```python
from build123d import *

# Parameters (mm, degrees)
BOSS_EXTRUDE1_DEPTH = 150


with BuildPart() as part:
    # Sketch1 → Boss-Extrude1 (new body)
    with BuildSketch(Plane.XY):
        with BuildLine():
            Line((12.999999999, 14.999999999), (10.499999999, 14.999999999))
            Line((10.499999999, 14.999999999), (9.999999999, 14.499999999))
            Line((9.999999999, 14.499999999), (9.5, 14.999999999))
            Line((9.5, 14.999999999), (4.5, 14.999999999))
            Line((4.5, 14.999999999), (4.5, 14.5))
            Line((4.5, 14.5), (4, 14.5))
            Line((4, 14.5), (4, 12.200000005))
            Line((4, 12.200000005), (7.999999994, 12.200000005))
            ThreePointArc((7.999999994, 12.200000005), (8.923879532, 11.582683434), (8.707106779, 10.492893215))
            Line((8.707106779, 10.492893215), (4.214213564, 6))
            Line((4.214213564, 6), (0.312520901, 6))
            Line((0.312520901, 6), (0, 5.7))
            Line((0, 5.7), (-0.312520903, 6))
            Line((-0.312520903, 6), (-4.214213564, 6))
            Line((-4.214213564, 6), (-8.70710678, 10.492893215))
            ThreePointArc((-8.70710678, 10.492893215), (-8.923879532, 11.582683434), (-7.999999995, 12.200000005))
            Line((-7.999999995, 12.200000005), (-4, 12.200000005))
            Line((-4, 12.200000005), (-4, 14.5))
            Line((-4, 14.5), (-4.5, 14.5))
            Line((-4.5, 14.5), (-4.5, 14.999999999))
            Line((-4.5, 14.999999999), (-9.500000003, 14.999999999))
            Line((-9.500000003, 14.999999999), (-10.000000002, 14.499999999))
            Line((-10.000000002, 14.499999999), (-10.500000001, 14.999999999))
            Line((-10.500000001, 14.999999999), (-13, 14.999999999))
            ThreePointArc((-13, 14.999999999), (-14.414213562, 14.414213561), (-15, 12.999999999))
            Line((-15, 12.999999999), (-15, 10.5))
            Line((-15, 10.5), (-14.500000001, 10.000000001))
            Line((-14.500000001, 10.000000001), (-15, 9.500000001))
            Line((-15, 9.500000001), (-15, 4.5))
            Line((-15, 4.5), (-14.5, 4.5))
            Line((-14.5, 4.5), (-14.5, 4))
            Line((-14.5, 4), (-12.200000005, 4))
            Line((-12.200000005, 4), (-12.200000005, 7.999999994))
            ThreePointArc((-12.200000005, 7.999999994), (-11.582683434, 8.923879532), (-10.492893215, 8.707106779))
            Line((-10.492893215, 8.707106779), (-6, 4.214213564))
            Line((-6, 4.214213564), (-6, 0.312520901))
            Line((-6, 0.312520901), (-5.7, 0))
            Line((-5.7, 0), (-6, -0.312520903))
            Line((-6, -0.312520903), (-6, -4.214213564))
            Line((-6, -4.214213564), (-10.492893215, -8.70710678))
            ThreePointArc((-10.492893215, -8.70710678), (-11.582683434, -8.923879532), (-12.200000005, -7.999999995))
            Line((-12.200000005, -7.999999995), (-12.200000005, -4))
            Line((-12.200000005, -4), (-14.5, -4))
            Line((-14.5, -4), (-14.5, -4.5))
            Line((-14.5, -4.5), (-15, -4.5))
            Line((-15, -4.5), (-15, -9.500000001))
            Line((-15, -9.500000001), (-14.500000001, -10.000000001))
            Line((-14.500000001, -10.000000001), (-15, -10.5))
            Line((-15, -10.5), (-15, -13))
            ThreePointArc((-15, -13), (-14.414213562, -14.414213562), (-13, -15))
            Line((-13, -15), (-10.489897949, -15))
            Line((-10.489897949, -15), (-9.989897949, -14.5))
            Line((-9.989897949, -14.5), (-9.500000001, -15))
            Line((-9.500000001, -15), (-4.5, -15))
            Line((-4.5, -15), (-4.5, -14.5))
            Line((-4.5, -14.5), (-4, -14.5))
            Line((-4, -14.5), (-4, -12.200000005))
            Line((-4, -12.200000005), (-7.999999995, -12.200000005))
            ThreePointArc((-7.999999995, -12.200000005), (-8.923879532, -11.582683434), (-8.70710678, -10.492893215))
            Line((-8.70710678, -10.492893215), (-4.214213564, -6))
            Line((-4.214213564, -6), (-0.312520901, -6))
            Line((-0.312520901, -6), (0, -5.7))
            Line((0, -5.7), (0.312520903, -6))
            Line((0.312520903, -6), (4.214213564, -6))
            Line((4.214213564, -6), (8.70710678, -10.492893215))
            ThreePointArc((8.70710678, -10.492893215), (8.923879532, -11.582683434), (7.999999995, -12.200000005))
            Line((7.999999995, -12.200000005), (4, -12.200000005))
            Line((4, -12.200000005), (4, -14.5))
            Line((4, -14.5), (4.5, -14.5))
            Line((4.5, -14.5), (4.5, -15))
            Line((4.5, -15), (9.500000001, -15))
            Line((9.500000001, -15), (10.000000001, -14.500000001))
            Line((10.000000001, -14.500000001), (10.5, -15))
            Line((10.5, -15), (12.999999999, -15))
            ThreePointArc((12.999999999, -15), (14.414213561, -14.414213562), (14.999999999, -13))
            Line((14.999999999, -13), (14.999999999, -10.500000001))
            Line((14.999999999, -10.500000001), (14.499999999, -10.000000002))
            Line((14.499999999, -10.000000002), (14.999999999, -9.500000002))
            Line((14.999999999, -9.500000002), (14.999999999, -4.5))
            Line((14.999999999, -4.5), (14.5, -4.5))
            Line((14.5, -4.5), (14.5, -4))
            Line((14.5, -4), (12.200000005, -4))
            Line((12.200000005, -4), (12.200000005, -7.999999995))
            ThreePointArc((12.200000005, -7.999999995), (11.582683434, -8.923879532), (10.492893215, -8.70710678))
            Line((10.492893215, -8.70710678), (6, -4.214213564))
            Line((6, -4.214213564), (6, -0.312520901))
            Line((6, -0.312520901), (5.7, 0))
            Line((5.7, 0), (6, 0.312520903))
            Line((6, 0.312520903), (6, 4.214213564))
            Line((6, 4.214213564), (10.492893215, 8.70710678))
            ThreePointArc((10.492893215, 8.70710678), (11.582683434, 8.923879532), (12.200000005, 7.999999995))
            Line((12.200000005, 7.999999995), (12.200000005, 4))
            Line((12.200000005, 4), (14.5, 4))
            Line((14.5, 4), (14.5, 4.5))
            Line((14.5, 4.5), (14.999999999, 4.5))
            Line((14.999999999, 4.5), (14.999999999, 9.5))
            Line((14.999999999, 9.5), (14.499999999, 9.999999999))
            Line((14.499999999, 9.999999999), (14.999999999, 10.499999999))
            Line((14.999999999, 10.499999999), (14.999999999, 12.999999999))
            ThreePointArc((14.999999999, 12.999999999), (14.414213561, 14.414213561), (12.999999999, 14.999999999))
        make_face()
        with BuildLine():
            Line((-2.902349714, 1.770978864), (-4.808326112, 3.676955262))
            Line((-4.808326112, 3.676955262), (-3.676955262, 4.808326112))
            Line((-3.676955262, 4.808326112), (-1.770978864, 2.902349714))
            ThreePointArc((-1.770978864, 2.902349714), (0, 3.4), (1.770978864, 2.902349714))
            Line((1.770978864, 2.902349714), (3.676955262, 4.808326112))
            Line((3.676955262, 4.808326112), (4.808326112, 3.676955262))
            Line((4.808326112, 3.676955262), (2.902349714, 1.770978864))
            ThreePointArc((2.902349714, 1.770978864), (3.4, 0), (2.902349714, -1.770978864))
            Line((2.902349714, -1.770978864), (4.808326112, -3.676955262))
            Line((4.808326112, -3.676955262), (3.676955262, -4.808326112))
            Line((3.676955262, -4.808326112), (1.770978864, -2.902349714))
            ThreePointArc((1.770978864, -2.902349714), (0, -3.4), (-1.770978864, -2.902349714))
            Line((-1.770978864, -2.902349714), (-3.676955262, -4.808326112))
            Line((-3.676955262, -4.808326112), (-4.808326112, -3.676955262))
            Line((-4.808326112, -3.676955262), (-2.902349714, -1.770978864))
            ThreePointArc((-2.902349714, -1.770978864), (-3.4, 0), (-2.902349714, 1.770978864))
        make_face(mode=Mode.SUBTRACT)
    extrude(amount=BOSS_EXTRUDE1_DEPTH)


solid = part.part
```
CAD build for the part. Positions are in the model's coordinates, mm. A direction names the side the tool comes from. Round coordinates to 2 decimals unless told otherwise and drop trailing zeros. One line per question, with ' | ' between items.
1. Probe L1, parallel to Y at x = -13, z = 27.5; L2, parallel to Y at x = -11.25, z = 45.5; L3, parallel to Y at x = -5, z = 138. List the from-to ranges inside material, lowest first. Write a range as from..to.
Working result:
L1: -15..-4, 4..15 | L2: -15..-9, 9..15 | L3: -15..-12.2, -6.79..6.79, 12.2..15
2. Mould opens along X. For faces 3 (the flat face through (-15, -12, 74)), 4 (the flat face through (2, 6, 74)), 5 (the flat face through (15, -12, 74)) say: pulls with the +X half, pulls with the -X half, needs draft (parallel to the pull), parting line crosses it, or undercut.
Working result:
face 3: pulls with the -X half | face 4: undercut | face 5: pulls with the +X half
3. Pin check, flat tips, straight feed: pin 1 Ø6 at (x, z) = (2.5, 69) entering from +Y; pin 2 Ø2 at (y, z) = (2.5, 101.5) entering from +X; pin 3 Ø0.5 at (x, z) = (15, 69.5) entering from -Y; pin 4 Ø2 at (y, z) = (-2, 77) entering from -X. Stop position of each tip, or through.
Working result:
pin 1: y = 15 | pin 2: x = 6 | pin 3: y = -13.97 | pin 4: x = -6
4. Which spindle directions (+Z, -Z, +X, -X, +Y, -Y) get a long thin tool onto all of the face, cutting with end or side? Do faces 1 (the flat face through (15, 7, 74)), 2 (the flat face through (-8.278, 6.492, 73.95)). Say none if no direction does.
Working result:
face 1: +Z, -Z, +X, +Y, -Y | face 2: +Z, -Z
